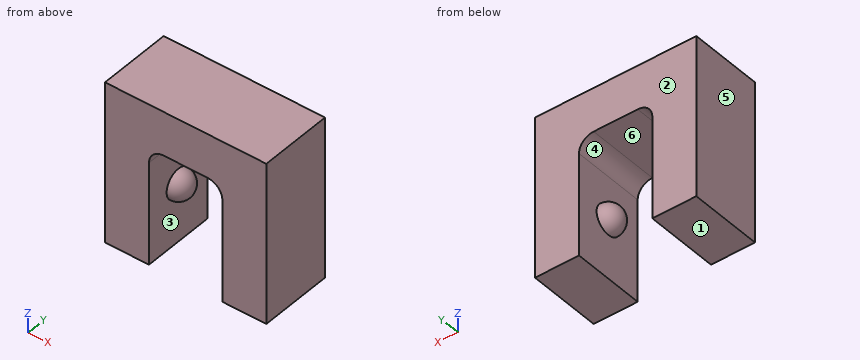
```python
from build123d import *

# Parameters (mm, degrees)
BOSS_EXTRUDE1_DEPTH = 5
FILLET1_R           = 1


with BuildPart() as part:
    # Sketch1 → Boss-Extrude1 (new body)
    with BuildSketch(Plane(origin=(0, 0, 0), x_dir=(1, 0, 0), z_dir=(0, 1, 0))):
        Polygon((-5.5, 5.5), (-5.5, -5.5), (5.5, -5.5), (5.5, 5.5), (2.5, 5.5), (2.5, 2.5), (2.5, -2.5), (-2.5, -2.5), (-2.5, 2.5), (-2.5, 5.5), align=None)
    extrude(amount=BOSS_EXTRUDE1_DEPTH)

    # Sketch2 → Revolve1 (revolve)
    with BuildSketch(Plane(origin=(-2.5, 0, 0), x_dir=(0, 0, -1), z_dir=(1, 0, 0))):
        with BuildLine():
            Line((2.5, 2.5), (0.5, 2.5))
            ThreePointArc((0.5, 2.5), (1.5, 1.5), (2.5, 2.5))
        make_face()
    revolve1 = revolve(axis=Axis((-2.5, 2.5, -5.5), (0, 0, 1)))

    # Mirror1: Revolve1 across plane
    add(revolve1.mirror(Plane(origin=(0, 0, 0), x_dir=(0, 0, 1), z_dir=(1, 0, 0))))

    # Fillet1
    fillet1_edges = [part.edges().sort_by_distance(p)[0] for p in [
        (-2.5, 2.5, 2.5),
        (2.5, 2.5, 2.5),
    ]]
    fillet(fillet1_edges, radius=FILLET1_R)


solid = part.part
```
Read the model definition and answer for the solid it produces. Units are mm, in the model's axes. Face numbers are marked on the shaded views. A direction names the side the tool comes from. Round coordinates to 2 decimals unless told otherwise and drop trailing zeros. Write each loop counter-clockwise with the first axis right and the second up, starting at its lowest first coordinate (ties: lowest second). Pieces come first, ordered by that corner, then holes. Notation, with made-up numbers: (-35.75, 10) -> (-12.75, 10) arc R29 ccw to (-12.75, 33) -> close; hole circle Ø3 at (39.5, 31.25). An arc over 180 degrees is marked (long way). Answer in a Markdown table with one row per item. Add a question column.
1) Find section A-A, the plane z = 0. Determine the outline of the cut face in (x, y), and give its area (3 significant figures).
2) Find section C-C, the plane x = -2. Determine the outline of the cut face in (y, z), and give its area (3 significant figures).
3) Determine the mould class of the marked faces 1, 2 and 3 for opening direction Z: pulls with the +Z half, pulls with the -Z half, needs draft (parallel to the pull), parting line crosses it, or undercut.
4) Consider line 1 (X direction, y = 4.1, z = -4.5); line 2 (Z direction, x = 0.75, y = 4.35); line 3 (Z direction, x = -2.25, y = 3.35). Determine where each line is inside the solid, lowest interval first.
5) Given P1, Ø4, axis at x = 0, z = -0.5, coming from the -Y side, flat-ended and moving along its own axis, determine where the tip first touches the part or whether it passes through.
6) Which of the six approach directions +Z, -Z, +X, -X, +Y, -Y give full straight-line access (tool end or side, diameter ignored) to the marked faces 4, 5 and 6?
7) Find section D-D, the plane y = 1.9. Determine the outline of the cut face in (x, z), and give its area (3 significant figures).
8) Find section B-B, the plane y = 4. Determine the outline of the cut face in (x, z).
Findings below:
| question | item | result |
|---|---|---|
| 1 | outline | (-5.5, 0) -> (-2.5, 0) -> (-2.5, 5) -> (-5.5, 5) -> close; (2.5, 0) -> (5.5, 0) -> (5.5, 5) -> (2.5, 5) -> close |
| 1 | area | 30.0 mm² |
| 2 | outline | (0, 2.37) -> (5, 2.37) -> (5, 5.5) -> (0, 5.5) -> close; circle Ø1.73 at (2.5, -1.5) |
| 2 | area | 18.0 mm² |
| 3 | face 1 | pulls with the -Z half |
| 3 | face 2 | needs draft |
| 3 | face 3 | undercut |
| 4 | line 1 | -5.5 to -2.5, 2.5 to 5.5 |
| 4 | line 2 | 2.5 to 5.5 |
| 4 | line 3 | -1.96 to -1.04, 2.16 to 5.5 |
| 5 | P1 | y = 1.78 |
| 6 | face 4 | +Y, -Y |
| 6 | face 5 | +Z, -Z, -X, +Y, -Y |
| 6 | face 6 | -Z, +Y, -Y |
| 7 | outline | (-5.5, -5.5) -> (-2.5, -5.5) -> (-2.5, -2.3) arc R0.8 ccw to (-2.5, -0.7) -> (-2.5, 1.5) arc R1 cw to (-1.5, 2.5) -> (1.5, 2.5) arc R1 cw to (2.5, 1.5) -> (2.5, -0.7) arc R0.8 ccw to (2.5, -2.3) -> (2.5, -5.5) -> (5.5, -5.5) -> (5.5, 5.5) -> (-5.5, 5.5) -> close |
| 7 | area | 83.4 mm² |
| 8 | outline | (-5.5, -5.5) -> (-2.5, -5.5) -> (-2.5, 1.5) arc R1 cw to (-1.5, 2.5) -> (1.5, 2.5) arc R1 cw to (2.5, 1.5) -> (2.5, -5.5) -> (5.5, -5.5) -> (5.5, 5.5) -> (-5.5, 5.5) -> close |
